Solid Edge part; units mm, degrees
sketch "Sketch1" plane through (0, 0, 0) normal (0, 0, 1) x (1, 0, 0)
  line L0 (-60.5, -14) -> (60.5, -14)
  line L1 (60.5, -14) -> (60.5, 14)
  line L2 (60.5, 14) -> (-60.5, 14)
  line L3 (-60.5, 14) -> (-60.5, -14)
extrude "Protrusion1" add sketch "Sketch1" against normal blind 40
sketch "Sketch2" plane through (0, -14, -20) normal (0, -1, 0) x (1, 0, 0)
  line L0 (60.5, 20) -> (42, 20)
  line L1 (42, 20) -> (42, 11.5)
  line L2 (42, 11.5) -> (60.5, 11.5)
  line L3 (60.5, 11.5) -> (60.5, 20)
  line L4 (-60.5, 11.5) -> (-42, 11.5)
  line L5 (-42, 11.5) -> (-42, 20)
  line L6 (-42, 20) -> (-60.5, 20)
  line L7 (-60.5, 20) -> (-60.5, 11.5)
extrude "ExtrudedCutout_1" cut sketch "Sketch2" against normal blind 28
extrude "Cutout1" [suppressed]
sketch "Sketch3" plane through (0, 11.075, 0) normal (0, 0, 1) x (1, 0, 0)
  line L0 (60.5, -2.925) -> (60.5, 0)
  line L1 (60.5, 0) -> (42, -2.925)
  line L2 (42, -2.925) -> (60.5, -2.925)
  line L3 (60.5, -19.225) -> (60.5, -22.125)
  line L4 (60.5, -22.125) -> (42, -19.225)
  line L5 (42, -19.225) -> (60.5, -19.225)
  line L6 (-60.5, -2.925) -> (-60.5, 0)
  line L7 (-60.5, 0) -> (-42, -2.925)
  line L8 (-42, -2.925) -> (-60.5, -2.925)
  line L9 (-60.5, -19.225) -> (-60.5, -22.15)
  line L10 (-60.5, -22.15) -> (-42, -19.225)
  line L11 (-42, -19.225) -> (-60.5, -19.225)
extrude "ExtrudedCutout_4" cut sketch "Sketch3" against normal blind 33
sketch "Sketch4" plane through (0, 0, 0) normal (0, 0, 1) x (1, 0, 0)
  line L0 (-60.5, -8.3) -> (60.5, -8.3)
  line L1 (60.5, -8.3) -> (60.5, 8.3)
  line L2 (60.5, 8.3) -> (-60.5, 8.3)
  line L3 (-60.5, 8.3) -> (-60.5, -8.3)
extrude "ExtrudedCutout_5" cut sketch "Sketch4" against normal blind 33
chamfer "Chamfer_2" distance 3 distance2 18 1 edges at (-60.5, 0, -33) measured on face at (-60.5, 9.6133, -34.435)
chamfer "Chamfer_3" distance 3 distance2 18 1 edges at (60.5, 0.0125, -33) measured on face at (60.5, -9.6133, -34.435)
sketch "Sketch5" plane through (0, -14, -20) normal (0, -1, 0) x (1, 0, 0)
  line L0 (-36.5, 20) -> (-42, 11.5)
  line L1 (-42, 11.5) -> (-42, 20)
  line L2 (-42, 20) -> (-36.5, 20)
  line L3 (36.5, 20) -> (42, 11.5)
  line L4 (42, 11.5) -> (42, 20)
  line L5 (42, 20) -> (36.5, 20)
extrude "ExtrudedCutout_6" cut sketch "Sketch5" against normal blind 40
chamfer "Chamfer_4" distance 3.5 angle 45 1 edges at (60.5, -12.525, -8.5)
chamfer "Chamfer_5" distance 3.5 angle 45 3 edges at (-60.5, -12.5375, -8.5) (-60.5, 12.5375, -8.5) (60.5, 12.5375, -8.5)
The listing builds one solid part. Answer for the finished solid, in the listing's coordinates (mm). A direction names the side the tool comes from. Round coordinates to 2 decimals unless told otherwise and drop trailing zeros. Order: outer loops, then holes, each group sorted by start corner. A loop starts at its lowest first (then second) coordinate and runs counter-clockwise, first axis right, second up. Notation, with made-up numbers: (61.25, 41) -> (74.25, 41) arc R25 ccw to (74.25, 60) -> close; hole circle Ø2 at (40, 18). An arc over 180 degrees is marked (long way). Put each result on its own line as item: value.
Q1. Each of these flat-tipped pins is pushed along its axis until it touches: P1, Ø6, axis at y = -2.5, z = -7.5, coming from the -X side; P2, Ø1.7, axis at x = 50.5, y = -11, coming from the +Z side; P3, Ø10, axis at y = 6.5, z = -32.5, coming from the -X side. Where does it stop, or does it pass through?
Results list:
P1: through
P2: z = -8.5
P3: x = -60.5
Q2. Section B-B, the plane x = -22 is taken. Write down the section's boundary in (y, z).
Results list:
outline: (-14, -40) -> (14, -40) -> (14, 0) -> (8.3, 0) -> (8.3, -33) -> (-8.3, -33) -> (-8.3, 0) -> (-14, 0) -> close
Q3. Consider line 1 along Y through (x, z) = (-41, -11); line 2 along Z through (x, y) = (-42.5, 7.75); line 3 along Z through (x, y) = (-44.5, -9.75). Determine where each line is inside the solid, lowest interval first.
Results list:
line 1: -14 to -8.3, 8.3 to 14
line 2: -40 to -33
line 3: -40 to -8.5
Q4. Which of the six approach directions +Z, -Z, +X, -X, +Y, -Y give full straight-line access (tool end or side, diameter ignored) to faces 1 (the flat face through (-51.8, -9.7, -22.1)), 2 (the flat face through (-50, 12, -8.5)), 3 (the flat face through (49, 12, -8.5)), 4 (the flat face through (51.37, 0.17, -34.48)), 5 (the flat face through (-60.5, -2, -36.3))?
Results list:
face 1: +Z, -X
face 2: +Z, -X, +Y, -Y
face 3: +Z, +X, +Y, -Y
face 4: +Z, +X
face 5: +Z, -Z, -X, +Y, -Y
Q5. Determine the mould class of faces 6 (the flat face through (49, -12, -8.5)), 7 (the flat face through (1, 14, -20)), 8 (the flat face through (-51.8, 9.7, -22.1)) for opening direction Y: pulls with the +Y half, pulls with the -Y half, needs draft (parallel to the pull), parting line crosses it, or undercut.
Results list:
face 6: needs draft
face 7: pulls with the +Y half
face 8: undercut
Q6. Section C-C, the plane y = -7 is taken. Write down the section's boundary in (x, z).
Results list:
outline: (-60.5, -40) -> (60.5, -40) -> (60.5, -36) -> (42.5, -33) -> (-42.5, -33) -> (-60.5, -36) -> close
Q7. Section A-A, the plane z = -31 is taken. Write down the section's boundary in (x, y) (3 decimals), and give its area (3 significant figures).
Results list:
outline: (-60.5, -14) -> (60.5, -14) -> (60.5, -11.05) -> (42.957, -8.3) -> (-42.949, -8.3) -> (-60.5, -11.075) -> close; (-60.5, 11.075) -> (-42.949, 8.3) -> (42.949, 8.3) -> (60.5, 11.075) -> (60.5, 14) -> (-60.5, 14) -> close
area: 1,280 mm^2
Q8. Section D-D, the plane x = 50 is taken. Write down the section's boundary in (y, z).
Results list:
outline: (-14, -40) -> (14, -40) -> (14, -8.5) -> (9.41, -8.5) -> (9.41, -34.25) -> (-9.4, -34.25) -> (-9.4, -8.5) -> (-14, -8.5) -> close
